from build123d import *

# Parameters (mm, degrees)
F0_R           = 19.05
F1_DEPTH       = 12.7
F2_R           = 19.05
F3_DEPTH       = 50.8
F5_DEPTH       = 31.75
F7_DEPTH       = 12.7
F15_DEPTH      = 2.54
F15_DEPTH_BACK = 12.7
F18_W          = 25.4
F18_H          = 25.4
F19_DEPTH      = 2.54
F22_DEPTH      = 6.35


# Not quite as in the source:
# - after a boolean that leaves OpenCascade's solid faulty, fix() repairs it
# - a feature of the source that left no trace in its solid (it failed there, or was rolled back) is left out


with BuildPart() as f1:
    # F0 (on Top) → F1 (new body)
    with BuildSketch(Plane.XY):
        with BuildLine():
            Line((82.55, 6.35), (82.55, 47.8529547439))
            ThreePointArc((82.55, 47.8529547439), (87.8105122421, 87.8105122421), (47.8529547439, 82.55))
            Line((47.8529547439, 82.55), (0, 82.55))
            Line((0, 82.55), (-47.8529547439, 82.55))
            ThreePointArc((-47.8529547439, 82.55), (-87.8105122421, 87.8105122421), (-82.55, 47.8529547439))
            Line((-82.55, 47.8529547439), (-82.55, 6.35))
            Line((-82.55, 6.35), (-82.55, 0))
            Line((-82.55, 0), (-82.55, -6.35))
            Line((-82.55, -6.35), (-82.55, -47.8529547439))
            ThreePointArc((-82.55, -47.8529547439), (-87.8105122421, -87.8105122421), (-47.8529547439, -82.55))
            Line((-47.8529547439, -82.55), (0, -82.55))
            Line((0, -82.55), (47.8529547439, -82.55))
            ThreePointArc((47.8529547439, -82.55), (87.8105122421, -87.8105122421), (82.55, -47.8529547439))
            Line((82.55, -47.8529547439), (82.55, -6.35))
            Line((82.55, -6.35), (82.55, 0))
            Line((82.55, 0), (82.55, 6.35))
        make_face()
        with Locations((-69.85, -69.85)):
            Circle(F0_R, mode=Mode.SUBTRACT)
        with BuildLine():
            Line((-6.35, -69.85), (-44.45, -69.85))
            ThreePointArc((-44.45, -69.85), (-45.345713546, -63.1641982245), (-47.9696807387, -56.9499368597))
            Line((-47.9696807387, -56.9499368597), (-6.35, -15.3302561211))
            Line((-6.35, -15.3302561211), (-6.35, -69.85))
        make_face(mode=Mode.SUBTRACT)
        with BuildLine():
            Line((-69.85, -6.35), (-15.3302561211, -6.35))
            Line((-15.3302561211, -6.35), (-56.9499368597, -47.9696807387))
            ThreePointArc((-56.9499368597, -47.9696807387), (-63.1641982245, -45.345713546), (-69.85, -44.45))
            Line((-69.85, -44.45), (-69.85, -6.35))
        make_face(mode=Mode.SUBTRACT)
        with Locations((69.85, -69.85)):
            Circle(F0_R, mode=Mode.SUBTRACT)
        with BuildLine():
            ThreePointArc((47.9696807387, -56.9499368597), (45.345713546, -63.1641982245), (44.45, -69.85))
            Line((44.45, -69.85), (6.35, -69.85))
            Line((6.35, -69.85), (6.35, -15.3302561211))
            Line((6.35, -15.3302561211), (47.9696807387, -56.9499368597))
        make_face(mode=Mode.SUBTRACT)
        with BuildLine():
            Line((56.9499368597, -47.9696807387), (15.3302561211, -6.35))
            Line((15.3302561211, -6.35), (69.85, -6.35))
            Line((69.85, -6.35), (69.85, -44.45))
            ThreePointArc((69.85, -44.45), (63.1641982245, -45.345713546), (56.9499368597, -47.9696807387))
        make_face(mode=Mode.SUBTRACT)
        with BuildLine():
            Line((-56.9499368597, 47.9696807387), (-15.3302561211, 6.35))
            Line((-15.3302561211, 6.35), (-69.85, 6.35))
            Line((-69.85, 6.35), (-69.85, 44.45))
            ThreePointArc((-69.85, 44.45), (-63.1641982245, 45.345713546), (-56.9499368597, 47.9696807387))
        make_face(mode=Mode.SUBTRACT)
        with BuildLine():
            Line((-6.35, 69.85), (-6.35, 15.3302561211))
            Line((-6.35, 15.3302561211), (-47.9696807387, 56.9499368597))
            ThreePointArc((-47.9696807387, 56.9499368597), (-45.345713546, 63.1641982245), (-44.45, 69.85))
            Line((-44.45, 69.85), (-6.35, 69.85))
        make_face(mode=Mode.SUBTRACT)
        with Locations((-69.85, 69.85)):
            Circle(F0_R, mode=Mode.SUBTRACT)
        with BuildLine():
            Line((69.85, 6.35), (15.3302561211, 6.35))
            Line((15.3302561211, 6.35), (56.9499368597, 47.9696807387))
            ThreePointArc((56.9499368597, 47.9696807387), (63.1641982245, 45.345713546), (69.85, 44.45))
            Line((69.85, 44.45), (69.85, 6.35))
        make_face(mode=Mode.SUBTRACT)
        with BuildLine():
            Line((6.35, 15.3302561211), (6.35, 69.85))
            Line((6.35, 69.85), (44.45, 69.85))
            ThreePointArc((44.45, 69.85), (45.345713546, 63.1641982245), (47.9696807387, 56.9499368597))
            Line((47.9696807387, 56.9499368597), (6.35, 15.3302561211))
        make_face(mode=Mode.SUBTRACT)
        with Locations((69.85, 69.85)):
            Circle(F0_R, mode=Mode.SUBTRACT)
    extrude(amount=F1_DEPTH)

    # F2 (on face) → F3 (join)
    with BuildSketch(Plane.XY.offset(12.7)):
        with BuildLine():
            ThreePointArc((-69.85, -44.45), (-76.4240037456, -45.3154840123), (-82.55, -47.8529547439))
            ThreePointArc((-82.55, -47.8529547439), (-87.8105122421, -87.8105122421), (-47.8529547439, -82.55))
            ThreePointArc((-47.8529547439, -82.55), (-45.3154840123, -76.4240037456), (-44.45, -69.85))
            ThreePointArc((-44.45, -69.85), (-45.345713546, -63.1641982245), (-47.9696807387, -56.9499368597))
            ThreePointArc((-47.9696807387, -56.9499368597), (-51.8894877579, -51.8894877579), (-56.9499368597, -47.9696807387))
            ThreePointArc((-56.9499368597, -47.9696807387), (-63.1641982245, -45.345713546), (-69.85, -44.45))
        make_face()
        with Locations((-69.85, -69.85)):
            Circle(F2_R, mode=Mode.SUBTRACT)
        with BuildLine():
            ThreePointArc((95.25, 69.85), (76.4240037456, 94.3845159877), (47.8529547439, 82.55))
            ThreePointArc((47.8529547439, 82.55), (45.3154840123, 76.4240037456), (44.45, 69.85))
            ThreePointArc((44.45, 69.85), (45.345713546, 63.1641982245), (47.9696807387, 56.9499368597))
            ThreePointArc((47.9696807387, 56.9499368597), (51.8894877579, 51.8894877579), (56.9499368597, 47.9696807387))
            ThreePointArc((56.9499368597, 47.9696807387), (63.1641982245, 45.345713546), (69.85, 44.45))
            ThreePointArc((69.85, 44.45), (76.4240037456, 45.3154840123), (82.55, 47.8529547439))
            ThreePointArc((82.55, 47.8529547439), (91.8470452561, 57.15), (95.25, 69.85))
        make_face()
        with Locations((69.85, 69.85)):
            Circle(F2_R, mode=Mode.SUBTRACT)
    extrude(amount=F3_DEPTH)

    # F10 (on offset) → F11 (revolve)
    with BuildSketch(Plane.XZ.offset(69.85)):
        with BuildLine():
            Line((-76.2, 82.55), (-95.25, 63.5))
            Line((-95.25, 63.5), (-88.9, 63.5))
            Line((-88.9, 63.5), (-69.85, 82.55))
            Line((-69.85, 82.55), (-69.85, 85.1802561211))
            ThreePointArc((-69.85, 85.1802561211), (-73.2865952359, 84.496674827), (-76.2, 82.55))
        make_face()
    revolve(axis=Axis((-69.85, -69.85, 63.5), (0, 0, 1)))


with BuildPart() as f5:
    # F4 (on Right) → F5 (new body, symmetric)
    with BuildSketch(Plane.YZ):
        with BuildLine():
            ThreePointArc((0, 127), (8.9802561211, 130.7197438789), (12.7, 139.7))
            ThreePointArc((12.7, 139.7), (-8.9802561211, 148.6802561211), (0, 127))
        make_face()
    extrude(amount=F5_DEPTH, both=True)

    # F6 (on face) → F7 (join)
    with BuildSketch(Plane(origin=(-31.75, 0, 0), x_dir=(0, -1, 0), z_dir=(-1, 0, 0))):
        with BuildLine():
            ThreePointArc((1.818e-07, 152.4), (-8.9802560568, 148.6802561853), (-12.7, 139.7))
            ThreePointArc((-12.7, 139.7), (-8.9802561211, 130.7197438789), (0, 127))
            ThreePointArc((0, 127), (8.9802561211, 130.7197438789), (12.7, 139.7))
            ThreePointArc((12.7, 139.7), (8.9802561853, 148.6802560568), (1.818e-07, 152.4))
        make_face()
        with BuildLine():
            Line((-12.7, 152.4), (-12.7, 139.7))
            ThreePointArc((-12.7, 139.7), (-8.9802560568, 148.6802561853), (1.818e-07, 152.4))
            Line((1.818e-07, 152.4), (-12.7, 152.4))
        make_face()
        with BuildLine():
            ThreePointArc((0, 127), (-8.9802561211, 130.7197438789), (-12.7, 139.7))
            Line((-12.7, 139.7), (-12.7, 127))
            Line((-12.7, 127), (0, 127))
        make_face()
    extrude(amount=F7_DEPTH)

    # F8: F5 across plane


with BuildPart() as f5_1:
    add(f5.part)
    add(f5.part.mirror(Plane.YZ))


with BuildPart() as f12_1:
    # F12: instance of F1
    add(f1.part.mirror(Plane.XZ))


with BuildPart() as f1_1:
    add(f1.part)

    add(f12_1.part)  # F13 merges F12_1
    # F13: F1, F12_1 across plane
    add(f1.part.mirror(Plane.YZ))
    add(f12_1.part.mirror(Plane.YZ))

    add(f5_1.part)  # F15 merges F5
    # F14 (on face) → F15 (join, two sides)
    with BuildSketch(Plane(origin=(-44.45, 0, 0), x_dir=(0, -1, 0), z_dir=(-1, 0, 0))) as f15_sk:
        Polygon((12.7, 139.7), (12.7, 127), (69.85, 12.7), (82.55, 12.7), (12.7, 152.4), align=None)
    extrude(amount=F15_DEPTH)
    extrude(f15_sk.sketch, amount=-F15_DEPTH_BACK)

    add(f1_1.part.fix(), mode=Mode.REPLACE)


with BuildPart() as f16_1:
    # F16: instance of F1
    add(f1_1.part.mirror(Plane.YZ))


with BuildPart() as f1_2:
    add(f1_1.part)

    add(f16_1.part)  # F17 merges F16_1
    # F17: F1, F16_1 across plane
    add(f1_1.part.mirror(Plane.XZ))
    add(f16_1.part.mirror(Plane.XZ))

    # F18 (on face) → F19 (join)
    with BuildSketch(Plane(origin=(-44.45, 0, 0), x_dir=(0, -1, 0), z_dir=(-1, 0, 0))):
        with Locations((0, 139.7)):
            Rectangle(F18_W, F18_H)
    extrude(amount=F19_DEPTH)

    # F21 (on Front) → F22 (join, symmetric)
    with BuildSketch(Plane.XZ):
        Polygon((-31.75, 152.4), (-46.99, 152.4), (-82.55, 12.7), (-69.85, 12.7), (-31.75, 127), align=None)
    extrude(amount=F22_DEPTH, both=True)

    # F23: F1 across plane


with BuildPart() as f1_3:
    add(f1_2.part)
    add(f1_2.part.mirror(Plane.YZ))


solid = f1_3.part
Here's how the part is built. I have some questions about the finished solid (model axes, mm). A direction names the side the tool comes from. Give positions to 0.01 mm unless a question says otherwise; leave off trailing zeros. Loops run counter-clockwise (first coordinate to the right, second up) from the corner with the lowest first, then second, coordinate; pieces in that order, holes last. Notation, with made-up numbers: (-19, 11) -> (15, 11) arc R25 ccw to (15, 39) -> close; hole circle Ø9 at (-32, 16). An arc over 180 degrees is marked (long way). Answer as a JSON object with one key per item and string values. Group by question number.
Item 1: Thinking about a two-plate mould opening in X: for faces 1 (the flat face through (-64.52, -0.09, 83.53)), 2 (the conical face through (-72.623, 74.2, 77.392)), 3 (the flat face through (-57, -6.35, 78)), which applies, pulls with the +X half, pulls with the -X half, needs draft (parallel to the pull), parting line crosses it, or undercut?
Item 2: Imagine slicing it at A-A on x = 2.5. Write out the boundary of the cut face in (y, z).
Item 3: I need wall thicknesses on L1, parallel to Y at x = 63.5, z = 24.5; L2, parallel to Y at x = -76, z = 69; L3, parallel to X at y = -77.5, z = 63. Which ranges of each line are inside material? Lowest first, please.
Item 4: Will these pins go through, and if not, where does the flat tip stop? pin 1 (14 mm diameter, centred on y = 30.5, z = 4, fed in from +X); pin 2 (6 mm diameter, centred on x = 3.5, y = -41, fed in from +Z); pin 3 (5 mm diameter, centred on x = 39.5, y = 9.5, fed in from -Z); pin 4 (23 mm diameter, centred on y = -63, z = 106.5, fed in from +X).
Item 5: Imagine slicing it at C-C on y = -24. Write out the boundary of the cut face in (x, z).
Item 6: On a 3-axis mill with a long thin cutter (end or side, diameter ignored), from which of +Z, -Z, +X, -X, +Y, -Y can I reach the whole of each face in a straight line? I mean faces 4 (the flat face through (-42, 6.35, 6)), 5 (the flat face through (69.85, 26, 6)), 6 (the flat face through (-1, -82.55, 6)), 7 (the flat face through (39.477, 40.875, 70.65)). Say none if no direction works.
Item 7: Imagine slicing it at B-B on z = 71. Give the number of separate pieces and of enclosed holes in the cut face, then the cut area to 3 significant figures.
Answer list:
{
 "1": {"face 1": "pulls with the -X half", "face 2": "undercut", "face 3": "needs draft"},
 "2": {"outline": "(-82.55, 0) -> (82.55, 0) -> (82.55, 12.7) -> (-82.55, 12.7) -> close; circle Ø25.4 at (0, 139.7)"},
 "3": {"L1": "y = -94.44 to -87.81, -51.89 to -45.26, 45.26 to 51.89, 87.81 to 94.44", "L2": "y = -88.78 to -81.92, -57.78 to -50.92, 50.92 to 57.78, 81.92 to 88.78", "L3": "x = -94.07 to -87.3, -52.4 to -45.63, 45.63 to 52.4, 87.3 to 94.07"},
 "4": {"pin 1": "stops at x = 82.55", "pin 2": "stops at z = 12.7", "pin 3": "stops at z = 127", "pin 4": "passes through"},
 "5": {"outline": "(-82.55, 0) -> (-69.85, 0) -> (-69.85, 12.7) -> (-82.55, 12.7) -> close; (-46.99, 104.4) -> (-31.75, 104.4) -> (-31.75, 129.8) -> (-46.99, 129.8) -> close; (-32.98, 0) -> (-15.02, 0) -> (-15.02, 12.7) -> (-32.98, 12.7) -> close; (-6.35, 0) -> (6.35, 0) -> (6.35, 12.7) -> (-6.35, 12.7) -> close; (15.02, 0) -> (32.98, 0) -> (32.98, 12.7) -> (15.02, 12.7) -> close; (31.75, 104.4) -> (46.99, 104.4) -> (46.99, 129.8) -> (31.75, 129.8) -> close; (69.85, 0) -> (82.55, 0) -> (82.55, 12.7) -> (69.85, 12.7) -> close"},
 "6": {"face 4": "-Z", "face 5": "+Z, -Z", "face 6": "+Z, -Z, -Y", "face 7": "none"},
 "7": {"separate pieces": "10", "enclosed holes": "4", "area": "3,560 mm2"}
}
